from build123d import *

# Parameters (mm, degrees)
SKETCH1_W           = 20
SKETCH1_H           = 20
BOSS_EXTRUDE1_DEPTH = 3
SKETCH2_W           = 20
SKETCH2_H           = 20
BOSS_EXTRUDE2_DEPTH = 3
BOSS_EXTRUDE3_DEPTH = 2
BOSS_EXTRUDE4_DEPTH = 2


with BuildPart() as part:
    # Sketch1 → Boss-Extrude1 (new body)
    with BuildSketch(Plane(origin=(0, 0, 0), x_dir=(1, 0, 0), z_dir=(0, 1, 0))):
        Rectangle(SKETCH1_W, SKETCH1_H)
        with BuildLine():
            Line((-2.95, -1.45), (-2.95, 1.45))
            ThreePointArc((-2.95, 1.45), (0, 4.4), (2.95, 1.45))
            Line((2.95, 1.45), (2.95, -1.45))
            ThreePointArc((2.95, -1.45), (0, -4.4), (-2.95, -1.45))
        make_face(mode=Mode.SUBTRACT)
    extrude(amount=BOSS_EXTRUDE1_DEPTH)

    # Sketch2 → Boss-Extrude2 (add)
    with BuildSketch(Plane(origin=(0, 0, -10), x_dir=(-1, 0, 0), z_dir=(0, 0, -1))):
        with Locations((0, 10)):
            Rectangle(SKETCH2_W, SKETCH2_H)
        with BuildLine():
            Line((-2.95, 8.55), (-2.95, 11.45))
            ThreePointArc((-2.95, 11.45), (0, 14.4), (2.95, 11.45))
            Line((2.95, 11.45), (2.95, 8.55))
            ThreePointArc((2.95, 8.55), (0, 5.6), (-2.95, 8.55))
        make_face(mode=Mode.SUBTRACT)
    extrude(amount=-BOSS_EXTRUDE2_DEPTH)

    # Sketch3 → Boss-Extrude3 (add)
    with BuildSketch(Plane(origin=(10, 0, 0), x_dir=(0, 0, -1), z_dir=(1, 0, 0))):
        Polygon((7, 20), (-10, 3), (7, 3), align=None)
    extrude(amount=-BOSS_EXTRUDE3_DEPTH)

    # Sketch4 → Boss-Extrude4 (add)
    with BuildSketch(Plane.ZY.offset(10)):
        Polygon((-7, 20), (-7, 3), (10, 3), align=None)
    extrude(amount=-BOSS_EXTRUDE4_DEPTH)


solid = part.part
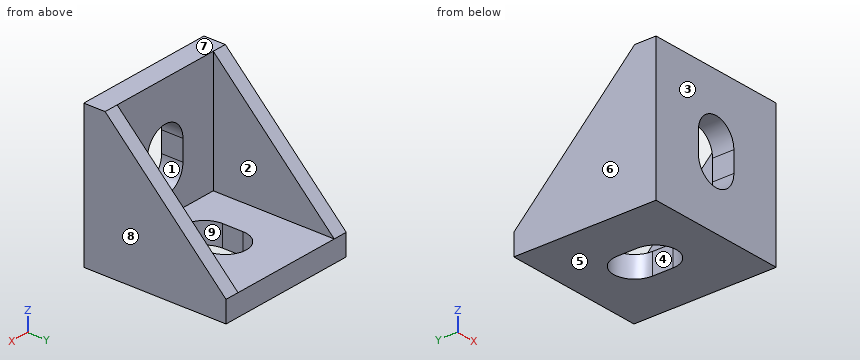
Read the model definition and answer for the solid it produces. Units are mm, in the model's axes. Face numbers are marked on the shaded views. A direction names the side the tool comes from. Round coordinates to 2 decimals unless told otherwise and drop trailing zeros. Write each loop counter-clockwise with the first axis right and the second up, starting at its lowest first coordinate (ties: lowest second). Pieces come first, ordered by that corner, then holes. Notation, with made-up numbers: (1, 64.25) - (39, 64.25) arc R11 ccw to (39, 82.25) - close; hole circle Ø10 at (81, 62). An arc over 180 degrees is marked (long way). Use a Markdown table: item, result.
(1) The part is cut by section D-D (z = 8). Write down the section's boundary in (x, y), then the cut area to 3 significant figures.
Reported:
| item | result |
|---|---|
| outline | (-10, 0) - (10, 0) - (10, 5) - (8, 5) - (8, 3) - (-8, 3) - (-8, 5) - (-10, 5) - close |
| area | 68.0 mm2 |
(2) The part is cut by section C-C (y = 2.5). Write down the section's boundary in (x, z), then the cut area to 3 significant figures.
Reported:
| item | result |
|---|---|
| outline | (-10, -10) - (10, -10) - (10, 10) - (-10, 10) - close; hole (-2.95, -1.45) arc R2.95 ccw to (2.95, -1.45) - (2.95, 1.45) arc R2.95 ccw to (-2.95, 1.45) - close |
| area | 356 mm2 |
(3) The part is cut by section B-B (x = 0). Write down the section's boundary in (y, z).
Reported:
| item | result |
|---|---|
| outline | (0, -10) - (5.6, -10) - (5.6, -7) - (3, -7) - (3, -4.4) - (0, -4.4) - close; (0, 4.4) - (3, 4.4) - (3, 10) - (0, 10) - close; (14.4, -10) - (20, -10) - (20, -7) - (14.4, -7) - close |
(4) The part is cut by section A-A (z = 0). Write down the section's boundary in (x, y), then the cut area to 3 significant figures.
Reported:
| item | result |
|---|---|
| outline | (-10, 0) - (-2.95, 0) - (-2.95, 3) - (-8, 3) - (-8, 13) - (-10, 13) - close; (2.95, 0) - (10, 0) - (10, 13) - (8, 13) - (8, 3) - (2.95, 3) - close |
| area | 82.3 mm2 |
(5) The mould has two halves that part along X. Classify the marked faces 6, 7, 8 and 9: released by +X, released by -X, zero draft, split by the parting line, or undercut.
Reported:
| item | result |
|---|---|
| face 6 | released by -X |
| face 7 | zero draft |
| face 8 | released by +X |
| face 9 | undercut |
(6) Each of these flat-tipped pins is pushed along its axis until it touches: pin 1 Ø4 at (x, z) = (6, -3.5) entering from -Y; pin 2 Ø8 at (x, z) = (-1.5, 4) entering from +Y. Where does it stop, or does it pass through?
Reported:
| item | result |
|---|---|
| pin 1 | y = 0 |
| pin 2 | y = 3 |
(7) Straight lines are drawn through the part: line 1 along X through (y, z) = (2.25, 0.5); line 2 along X through (y, z) = (8, 4.75); line 3 along Y through (x, z) = (-4.25, -5.75). For each, find the intervals that lie inside material, in ascending order. Write a range as [from, to].
Reported:
| item | result |
|---|---|
| line 1 | [-10, -2.95], [2.95, 10] |
| line 2 | [-10, -8], [8, 10] |
| line 3 | [0, 3] |
(8) Which of the six approach directions +Z, -Z, +X, -X, +Y, -Y give full straight-line access (tool end or side, diameter ignored) to the marked faces 1, 2, 3, 4 and 5?
Reported:
| item | result |
|---|---|
| face 1 | +Y, -Y |
| face 2 | +Z, +Y |
| face 3 | +Z, -Z, +X, -X, -Y |
| face 4 | +Z, -Z |
| face 5 | -Z, +X, -X, +Y, -Y |
